Read the model definition and answer for the solid it produces. Units are mm, in the model's axes. Face numbers are marked on the shaded views. A direction names the side the tool comes from. Give positions to 0.01 mm unless a question says otherwise; leave off trailing zeros. Order: outer loops, then holes, each group sorted by start corner. A loop starts at its lowest first (then second) coordinate and runs counter-clockwise, first axis right, second up. Notation, with made-up numbers: (48, -22.75) - (104, -22.75) arc R21 ccw to (104, -10.75) - close; hole circle Ø11 at (-31.5, 82). An arc over 180 degrees is marked (long way). Write item = value, one per line.
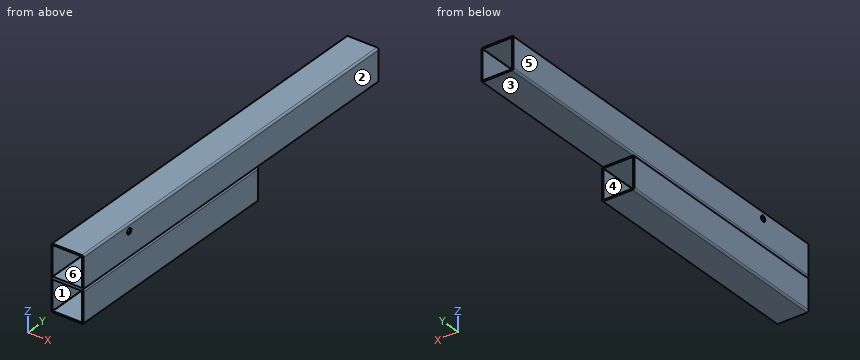
```python
from build123d import *

# Parameters (mm, degrees)
F1_DEPTH = 1100
F2_R     = 8
F3_DEPTH = 90.001
F4_W     = 450
F4_H     = 80
F4_H_2   = 5
F5_DEPTH = 90.001


with BuildPart() as f1:
    # F0 (on Front) → F1 (new body)
    with BuildSketch(Plane.XZ):
        with BuildLine():
            ThreePointArc((45, 40), (43.5355339059, 43.5355339059), (40, 45))
            Line((40, 45), (-40, 45))
            ThreePointArc((-40, 45), (-43.5355339059, 43.5355339059), (-45, 40))
            Line((-45, 40), (-45, -40))
            ThreePointArc((-45, -40), (-43.5355339059, -43.5355339059), (-40, -45))
            Line((-40, -45), (40, -45))
            ThreePointArc((40, -45), (43.5355339059, -43.5355339059), (45, -40))
            Line((45, -40), (45, 40))
        make_face()
        with BuildLine():
            ThreePointArc((-41, 40), (-40.7071067812, 40.7071067812), (-40, 41))
            Line((-40, 41), (40, 41))
            ThreePointArc((40, 41), (40.7071067812, 40.7071067812), (41, 40))
            Line((41, 40), (41, -40))
            ThreePointArc((41, -40), (40.7071067812, -40.7071067812), (40, -41))
            Line((40, -41), (-40, -41))
            ThreePointArc((-40, -41), (-40.7071067812, -40.7071067812), (-41, -40))
            Line((-41, -40), (-41, 40))
        make_face(mode=Mode.SUBTRACT)
        with BuildLine():
            ThreePointArc((45, -50), (43.5355339059, -46.4644660941), (40, -45))
            Line((40, -45), (-40, -45))
            ThreePointArc((-40, -45), (-43.5355339059, -46.4644660941), (-45, -50))
            Line((-45, -50), (-45, -130))
            ThreePointArc((-45, -130), (-43.5355339059, -133.5355339059), (-40, -135))
            Line((-40, -135), (40, -135))
            ThreePointArc((40, -135), (43.5355339059, -133.5355339059), (45, -130))
            Line((45, -130), (45, -50))
        make_face()
        with BuildLine():
            ThreePointArc((-41, -50), (-40.7071067812, -49.2928932188), (-40, -49))
            Line((-40, -49), (40, -49))
            ThreePointArc((40, -49), (40.7071067812, -49.2928932188), (41, -50))
            Line((41, -50), (41, -130))
            ThreePointArc((41, -130), (40.7071067812, -130.7071067812), (40, -131))
            Line((40, -131), (-40, -131))
            ThreePointArc((-40, -131), (-40.7071067812, -130.7071067812), (-41, -130))
            Line((-41, -130), (-41, -50))
        make_face(mode=Mode.SUBTRACT)
    extrude(amount=-F1_DEPTH)

    # F2 (on face) → F3 (cut, through all)
    with BuildSketch(Plane.YZ.offset(45)):
        with Locations((170, 25)):
            Circle(F2_R)
    extrude(amount=-F3_DEPTH, mode=Mode.SUBTRACT)

    # F4 (on face) → F5 (cut, through all)
    with BuildSketch(Plane.YZ.offset(45)):
        with Locations((875, -90)):
            Rectangle(F4_W, F4_H)
        with Locations((875, -132.5)):
            Rectangle(F4_W, F4_H_2)
        with Locations((875, -47.5)):
            Rectangle(F4_W, F4_H_2)
    extrude(amount=-F5_DEPTH, mode=Mode.SUBTRACT)


solid = f1.part
```
1. For the marked faces 5 and 6, determine the directions among +Z, -Z, +X, -X, +Y, -Y from which every point of the face is accessible in a straight line to the end or side of a thin tool.
Recorded:
face_5 = +Z, -Z, -X, +Y, -Y
face_6 = +Y, -Y
2. Determine the mould class of the marked faces 1, 2, 3 and 4 for opening direction Z: +Z half, -Z half, draft (parallel to the pull), parting line (faces both ways), or undercut.
Recorded:
face_1 = undercut
face_2 = draft
face_3 = -Z half
face_4 = undercut
3. Section B-B (y = 208.5) is taken. Count the separate pieces of the cut face and the enclosed holes in it, and give its area (3 significant figures).
Recorded:
separate_pieces = 1
enclosed_holes = 2
area = 2,710 mm^2
4. Section C-C (x = 12) is taken. Determine the outline of the cut face in (y, z).
Recorded:
outline = (0, -135) - (650, -135) - (650, -131) - (0, -131) - close; (0, -49) - (650, -49) - (650, -45) - (1100, -45) - (1100, -41) - (0, -41) - close; (0, 41) - (1100, 41) - (1100, 45) - (0, 45) - close
5. Section D-D (y = 804) is taken. Determine the outline of the cut face in (x, z).
Recorded:
outline = (-45, -40) arc R5 ccw to (-40, -45) - (40, -45) arc R5 ccw to (45, -40) - (45, 40) arc R5 ccw to (40, 45) - (-40, 45) arc R5 ccw to (-45, 40) - close; hole (-41, -40) arc R1 ccw to (-40, -41) - (40, -41) arc R1 ccw to (41, -40) - (41, 40) arc R1 ccw to (40, 41) - (-40, 41) arc R1 ccw to (-41, 40) - close
6. A flat-ended cylindrical pin translates along its axis: pin 1 (2 mm diameter, centred on y = 736.5, z = -41.5, fed in from -X). Find the tip coordinate at first contact, or state that the pin passes through.
Recorded:
pin_1 = -44.97
7. Straight lines are drawn through the part: L1, parallel to Z at x = 34.5, y = 594; L2, parallel to X at y = 924, z = 21. For each, find the intervals that lie inside material, in ascending order. Write a range as [from, to].
Recorded:
L1 = [-135, -131], [-49, -41], [41, 45]
L2 = [-45, -41], [41, 45]
8. Section A-A (z = 8) is taken. Determine the outline of the cut face in (x, y), and give its area (3 significant figures).
Recorded:
outline = (-45, 0) - (-41, 0) - (-41, 1100) - (-45, 1100) - close; (41, 0) - (45, 0) - (45, 1100) - (41, 1100) - close
area = 8,800 mm^2
